```python
from build123d import *

# Parameters (mm, degrees)
SKETCH_1_W      = 16
SKETCH_1_H      = 10
EXTRUDE_1_DEPTH = 3
FILLET_1_R      = 2


with BuildPart() as part:
    # 草图1 → 凸台-拉伸1 (new body)
    with BuildSketch(Plane.XY):
        Polygon((-8, -5), (-8, -3.231128538), (-13.860388679, -6.893871462), (-18, -6.893871462), (-18, -9.893871462), (-13, -9.893871462), (-5.16980566, -5), align=None)
        Rectangle(SKETCH_1_W, SKETCH_1_H)
    extrude(amount=EXTRUDE_1_DEPTH)

    # 圆角1
    fillet_1_edges = [part.edges().sort_by_distance(p)[0] for p in [
        (-13, -9.893871462, 1.5),
        (-13.860388679, -6.893871462, 1.5),
        (-8, -3.231128538, 1.5),
        (-8, 5, 1.5),
        (8, 5, 1.5),
        (8, -5, 1.5),
        (-5.16980566, -5, 1.5),
    ]]
    fillet(fillet_1_edges, radius=FILLET_1_R)


solid = part.part
```
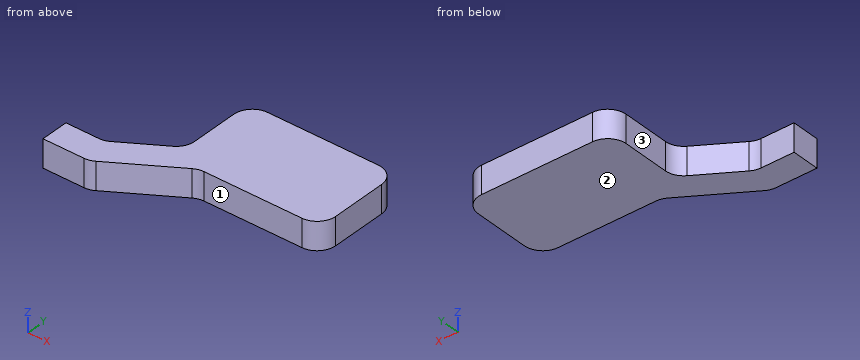
Input: part model. Units: mm. Frame: model coordinates. Face numbers are marked on the shaded views. A direction names the side the tool comes from. Give positions to 0.01 mm unless a question says otherwise; leave off trailing zeros. Order: outer loops, then holes, each group sorted by start corner. A loop starts at its lowest first (then second) coordinate and runs counter-clockwise, first axis right, second up.
1. Cut plane B-B (x = -15.25). Return loops of the section in (y, z).
Computed:
outline: (-9.89, 0) - (-6.89, 0) - (-6.89, 3) - (-9.89, 3) - close
2. Cut plane C-C (y = 0.25). Return loops of the section in (x, z).
Computed:
outline: (-8, 0) - (8, 0) - (8, 3) - (-8, 3) - close
3. Cut plane A-A (z = 0.95). Return loops of the section in (x, y).
Computed:
outline: (-18, -9.89) - (-13.57, -9.89) arc R2 ccw to (-12.51, -9.59) - (-5.66, -5.3) arc R2 cw to (-4.6, -5) - (6, -5) arc R2 ccw to (8, -3) - (8, 3) arc R2 ccw to (6, 5) - (-6, 5) arc R2 ccw to (-8, 3) - (-8, -2.12) arc R2 cw to (-8.94, -3.82) - (-13.37, -6.59) arc R2 cw to (-14.43, -6.89) - (-18, -6.89) - close
4. Line query: probe 1 along X at (y, z) = (2, 2.75); probe 2 along Y at (x, z) = (-0.25, 1.8); probe 3 along Y at (x, z) = (-15.5, 0.35). Output: solid intervals per line, ascending.
Computed:
probe 1: x = -8 to 8
probe 2: y = -5 to 5
probe 3: y = -9.89 to -6.89
5. Pin query (flat end, axial travel): pin 1 Ø1.5 at (x, z) = (1.5, 1.5) entering from -Y; pin 2 Ø5 at (x, y) = (-9, -8.5) entering from -Z; pin 3 Ø1.5 at (y, z) = (0.5, 1.5) entering from -X. Return the tip coordinate at first contact, or that it passes through.
Computed:
pin 1: stops at y = -5
pin 2: stops at z = 0
pin 3: stops at x = -8
6. Set-up query: the marked faces 1, 2 and 3. Return all of +Z, -Z, +X, -X, +Y, -Y with unobstructed straight access to the full face (end or side cutting, diameter ignored); none if empty.
Computed:
face 1: +Z, -Z, +X, -Y
face 2: -Z, +X, -X, +Y, -Y
face 3: +Z, -Z, -X, +Y
